For this review, take the finished solid that the model builds, in its own axes (mm). Face numbers are marked on the shaded views. A direction names the side the tool comes from. Coordinates: 2 decimals unless noted, no trailing zeros. Write each loop counter-clockwise with the first axis right and the second up, starting at its lowest first coordinate (ties: lowest second). Pieces come first, ordered by that corner, then holes. Notation, with made-up numbers: M 26.5,72.25 L 55.5,72.25 A23 cw 55.5,81.25 Z; hole C -11.75,23 d5. An arc over 180 degrees is marked long. Return JSON: item names as keys, results as strings.
```python
from build123d import *

# Parameters (mm, degrees)
F2_R    = 5
F3_SIZE = 2


with BuildPart() as f1:
    # F0 (on Front) → F1 (revolve)
    with BuildSketch(Plane.XZ):
        Polygon((-79.4498865843, -12.1671419008), (-79.4498865843, 132.3328580992), (-81.0498865843, 132.3328580992), (-88.9998865843, 126.2326085448), (-88.9998865843, 117.5993978977), (-114.3998865843, 30.7328580992), (-184.2498865843, 30.7328580992), (-184.2498865843, -10.5671419008), (-127.0998865843, -10.5671419008), (-127.0998865843, -12.1671419008), align=None)
    revolve(axis=Axis((165.0001134157, 0, 0.9622275829), (0, 0, -1)))

    # F2
    f2_edges = [f1.edges().sort_by_distance(p)[0] for p in [
        (514.250113, 0, 30.732858),
    ]]
    fillet(f2_edges, radius=F2_R)

    # F3
    f3_edges = [f1.edges().sort_by_distance(p)[0] for p in [
        (514.250113, 0, -10.567142),
    ]]
    chamfer(f3_edges, length=F3_SIZE)


solid = f1.part
```
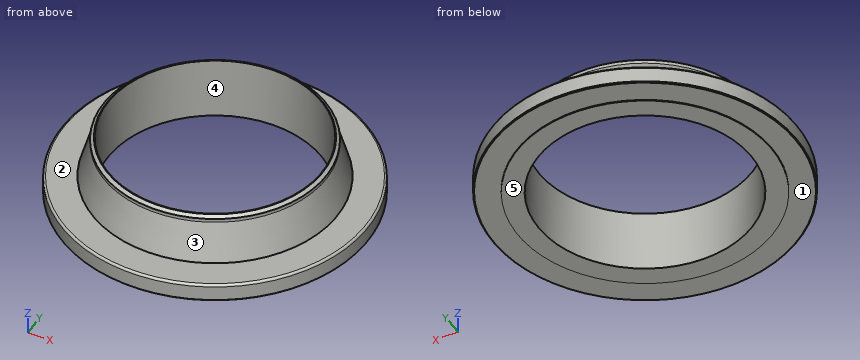
1. Wall thickness on L1, parallel to Z at x = 316, y = -274; L2, parallel to Y at x = 44.5, z = 80; L3, parallel to Y at x = 227.5, z = 118: over which ranges is each line inside the solid? List them lowest first. Write a range as from..to.
Checks:
{"L1": "-10.57..30.73", "L2": "-236.01..-212.69, 212.69..236.01", "L3": "-246.19..-236.33, 236.33..246.19"}
2. We need section B-B (z = 108.5). State the section outline as (x, y) points, plus the area to 3 significant figures.
Checks:
{"outline": "C 165,0 d513.32; hole C 165,0 d488.9", "area": "19,200 mm2"}
3. Draft analysis for pull direction X (two halves, no side actions). For the marked faces 3, 4 and 5, state which applies: +X half, -X half, draft (parallel to the pull), parting line (faces both ways), or undercut.
Checks:
{"face 3": "parting line", "face 4": "undercut", "face 5": "draft"}
4. For the marked faces 1 and 2, list the 3-axis set-ups (+Z, -Z, +X, -X, +Y, -Y) from which the entire face can be reached by the end or side of a thin tool; tool diameter is ignored.
Checks:
{"face 1": "-Z", "face 2": "+Z"}
5. Clearance check with flat-ended pins moving along their axes: pin 1 Ø4 at (y, z) = (202, 103) entering from +X; pin 2 Ø6 at (y, z) = (-74.5, 61.5) entering from +X; pin 3 Ø6 at (x, z) = (395.5, 13.5) entering from +Y. State where each tip first meets the part, or that it passes through.
Checks:
{"pin 1": "x = 328.58", "pin 2": "x = 426.18", "pin 3": "y = 264.99"}
6. We need section A-A (y = 0). State the section outline as (x, z) points, plus the area to 3 significant figures.
Checks:
{"outline": "M -184.25,-8.57 L -182.25,-10.57 L -127.1,-10.57 L -127.1,-12.17 L -79.45,-12.17 L -79.45,132.33 L -81.05,132.33 L -89,126.23 L -89,117.6 L -114.4,30.73 L -179.25,30.73 A5 ccw -184.25,25.73 Z; M 409.45,-12.17 L 457.1,-12.17 L 457.1,-10.57 L 512.25,-10.57 L 514.25,-8.57 L 514.25,25.73 A5 ccw 509.25,30.73 L 444.4,30.73 L 419,117.6 L 419,126.23 L 411.05,132.33 L 409.45,132.33 Z", "area": "12,900 mm2"}
7. We need section C-C (z = 43). State the section outline as (x, y) points, plus the area to 3 significant figures.
Checks:
{"outline": "C 165,0 d551.63; hole C 165,0 d488.9", "area": "51,300 mm2"}
